```python
from build123d import *

# Parameters (mm, degrees)
SKIZZE1_W                       = 16
SKIZZE1_H                       = 63
SKIZZE6_W                       = 14.056140901
SKIZZE6_H                       = 6
SCHNITT_LINEAR_AUSTRAGEN2_DEPTH = 2.9
SKIZZE8_W                       = 9.697943534
SKIZZE8_H                       = 4.605462576
VERRUNDUNG1_R                   = 2.7
SKIZZE9_W                       = 13.512274764
SKIZZE9_H                       = 9
SKIZZE11_W                      = 2.793838278
SKIZZE11_H                      = 24.477994545
SKIZZE12_W                      = 8.586499361
SKIZZE12_H                      = 1
VERRUNDUNG2_R                   = 1.5
VERRUNDUNG3_R                   = 1
VERRUNDUNG4_R                   = 1


with BuildPart() as part:
    # Skizze1 → Rotation1 (revolve)
    with BuildSketch(Plane(origin=(0, 0, 0), x_dir=(0, 0, -1), z_dir=(1, 0, 0))):
        with Locations((-18, -0.15056419)):
            Rectangle(SKIZZE1_W, SKIZZE1_H)
    revolve(axis=Axis((0, 31.34943581, 10), (0, -1, 0)))

    # Skizze6 → Schnitt-Rotation1 (revolve, cut)
    with BuildSketch(Plane.XY.offset(10), mode=Mode.PRIVATE) as schnitt_rotation1_sk:
        with Locations((-10.028070451, 28.34943581)):
            Rectangle(SKIZZE6_W, SKIZZE6_H)
    revolve(schnitt_rotation1_sk.sketch.rotate(Axis((0, 55, 10), (0, -1, 0)), 270), axis=Axis((0, 55, 10), (0, -1, 0)), mode=Mode.SUBTRACT)

    # Skizze7 → Schnitt-Linear austragen2 (cut)
    with BuildSketch(Plane.XZ.offset(31.65056419)):
        with BuildLine():
            Line((-10.583005244, 22), (10.583005244, 22))
            ThreePointArc((10.583005244, 22), (0, 26), (-10.583005244, 22))
        make_face()
        with BuildLine():
            ThreePointArc((16, 10), (14.966629547, 15.656854249), (12, 20.583005244))
            Line((12, 20.583005244), (12, -0.583005244))
            ThreePointArc((12, -0.583005244), (14.966629547, 4.343145751), (16, 10))
        make_face()
        with BuildLine():
            ThreePointArc((-10.583005244, -2), (0, -6), (10.583005244, -2))
            Line((10.583005244, -2), (-10.583005244, -2))
        make_face()
        with BuildLine():
            Line((-12, -0.583005244), (-12, 20.583005244))
            ThreePointArc((-12, 20.583005244), (-16, 10), (-12, -0.583005244))
        make_face()
    extrude(amount=-SCHNITT_LINEAR_AUSTRAGEN2_DEPTH, mode=Mode.SUBTRACT)

    # Skizze8 → Schnitt-Rotation2 (revolve, cut)
    with BuildSketch(Plane.XY.offset(10), mode=Mode.PRIVATE) as schnitt_rotation2_sk:
        with Locations((-13.848971767, -26.447832902)):
            Rectangle(SKIZZE8_W, SKIZZE8_H)
    revolve(schnitt_rotation2_sk.sketch.rotate(Axis((0, 55, 10), (0, -1, 0)), 270), axis=Axis((0, 55, 10), (0, -1, 0)), mode=Mode.SUBTRACT)

    # Verrundung1
    # the kernel refuses this fillet: 2.7 mm, written as the material it takes off along each edge
    with BuildSketch(Plane(origin=(-12, -34.598571865, 20.583005244), x_dir=(0.6886261541674549, 0, 0.72511655600775), z_dir=(0, 1, 0)), Plane(origin=(-10.583005244, -34.598571865, -2), x_dir=(-0.7251165560077487, 0, 0.6886261541674565), z_dir=(0, 1, 0)), Plane(origin=(10.583005244, -34.598571865, 22), x_dir=(0.72511655600775, 0, -0.6886261541674551), z_dir=(0, 1, 0)), Plane(origin=(12, -34.598571865, -0.583005244), x_dir=(-0.6886261541674555, 0, -0.7251165560077496), z_dir=(0, 1, 0))) as verrundung1_piece_1:
        with BuildLine():
            CenterArc((1.079707811, 2.698166172), VERRUNDUNG1_R, 226.478544781, 45.633288329)
            Line((-0.779582805, 0.740351471), (0, 0))
            ThreePointArc((0, 0), (0.589601535, -0.010867127), (1.17920307, 0))
        make_face()
    extrude(amount=8.796015351, mode=Mode.SUBTRACT)
    with BuildSketch(Plane(origin=(-12, -34.598571865, -0.583005244), x_dir=(0, 0, 1), z_dir=(0, 1, 0)), Plane(origin=(10.583005244, -34.598571865, -2), x_dir=(-1, 0, 0), z_dir=(0, 1, 0)), Plane(origin=(12, -34.598571865, 20.583005244), x_dir=(0, 0, -1), z_dir=(0, 1, 0))) as verrundung1_piece_2:
        with BuildLine():
            CenterArc((1.075113785, 2.7), VERRUNDUNG1_R, 224.366711671, 45.633288329)
            ThreePointArc((-0.855059669, 0.812030075), (-0.435013222, 0.398135104), (0, 0))
            Line((0, 0), (1.075113785, 0))
        make_face()
    extrude(amount=8.796015351, mode=Mode.SUBTRACT)
    with BuildSketch(Plane(origin=(-10.583005244, -34.598571865, 22), x_dir=(-0.7251165560077509, 0, -0.6886261541674541), z_dir=(0, 1, 0))) as verrundung1_piece_3:
        with BuildLine():
            CenterArc((1.079707811, -2.698166172), VERRUNDUNG1_R, 87.88816689, 45.633288329)
            Line((-0.779582805, -0.740351471), (0, 0))
            ThreePointArc((0, 0), (0.589601535, 0.010867127), (1.17920307, 0))
        make_face()
    extrude(amount=8.796015351, mode=Mode.SUBTRACT)

    # Skizze9 → Schnitt-Rotation3 (revolve, cut)
    with BuildSketch(Plane.XY.offset(10), mode=Mode.PRIVATE) as schnitt_rotation3_sk:
        with Locations((10.756137382, 11.84943581)):
            Rectangle(SKIZZE9_W, SKIZZE9_H)
    revolve(schnitt_rotation3_sk.sketch.rotate(Axis((0, 55, 10), (0, -1, 0)), 90), axis=Axis((0, 55, 10), (0, -1, 0)), mode=Mode.SUBTRACT)

    # Skizze11 → Schnitt-Rotation4 (revolve, cut)
    with BuildSketch(Plane.XY.offset(10), mode=Mode.PRIVATE) as schnitt_rotation4_sk:
        with Locations((-16.396919139, -4.411566918)):
            Rectangle(SKIZZE11_W, SKIZZE11_H)
    revolve(schnitt_rotation4_sk.sketch.rotate(Axis((0, 55, 10), (0, -1, 0)), 270), axis=Axis((0, 55, 10), (0, -1, 0)), mode=Mode.SUBTRACT)

    # Skizze12 → Schnitt-Rotation5 (revolve, cut)
    with BuildSketch(Plane.XY.offset(10), mode=Mode.PRIVATE) as schnitt_rotation5_sk:
        with Locations((-13.293249681, -16.15056419)):
            Rectangle(SKIZZE12_W, SKIZZE12_H)
    revolve(schnitt_rotation5_sk.sketch.rotate(Axis((0, 55, 10), (0, -1, 0)), 270), axis=Axis((0, 55, 10), (0, -1, 0)), mode=Mode.SUBTRACT)

    # Verrundung2
    verrundung2_edges = [part.edges().sort_by_distance(p)[0] for p in [
        (0, 25.34943581, -6),
    ]]
    fillet(verrundung2_edges, radius=VERRUNDUNG2_R)

    # Verrundung3
    verrundung3_edges = [part.edges().sort_by_distance(p)[0] for p in [
        (0, -16.65056419, -6),
        (0, -24.145101614, -6),
    ]]
    fillet(verrundung3_edges, radius=VERRUNDUNG3_R)

    # Verrundung4
    verrundung4_edges = [part.edges().sort_by_distance(p)[0] for p in [
        (0, 7.34943581, -5),
        (0, -15.65056419, -5),
    ]]
    fillet(verrundung4_edges, radius=VERRUNDUNG4_R)


solid = part.part
```
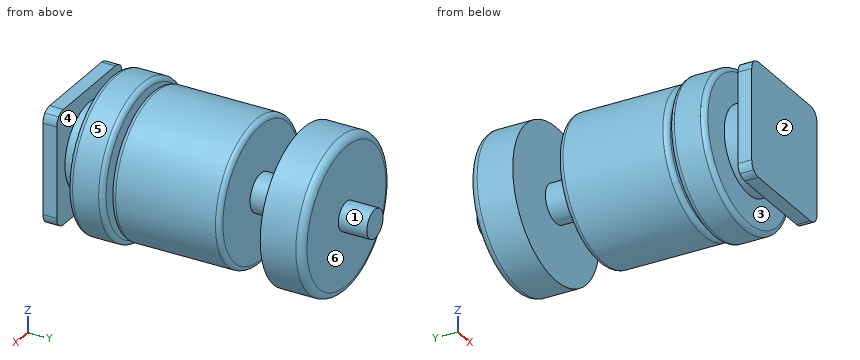
For this review, take the finished solid that the model builds, in its own axes (mm). Face numbers are marked on the shaded views. A direction names the side the tool comes from. Give positions to 0.01 mm unless a question says otherwise; leave off trailing zeros. Write each loop counter-clockwise with the first axis right and the second up, starting at its lowest first coordinate (ties: lowest second). Pieces come first, ordered by that corner, then holes. Notation, with made-up numbers: M 38,55 L 83,55 A36 cw 83,94 Z; hole C 60,29.5 d8. An arc over 180 degrees is marked long. Answer as a JSON object with one key per item and string values. Group by question number.
Item 1: Consider section A-A on y = -13. Write out the cut boundary in (x, z).
Item 2: Tool access review of the marked faces 1, 2 and 3: name each direction out of +Z, -Z, +X, -X, +Y, -Y from which nothing blocks a thin tool from reaching the whole face with its end or side.
Item 3: Consider section B-B on y = 19. Write out the cut boundary in (x, z).
Item 4: Draft analysis for pull direction Y (two halves, no side actions). For the marked faces 4, 5 and 6, state which applies: +Y half, -Y half, draft (parallel to the pull), parting line (faces both ways), or undercut.
Item 5: For pin 1 Ø2.5 at (x, y) = (0.5, -31) entering from -Z; pin 2 Ø1.4 at (y, z) = (-30.5, 11.5) entering from -X; pin 3 Ø3 at (x, y) = (1, -30.5) entering from +Z, all flat-tipped, find the tip position at first contact; note any pin that passes through.
Item 6: For probe 1 along Y at (x, z) = (-11, 7.5); probe 2 along Y at (x, z) = (3.5, -3); probe 3 along Y at (x, z) = (-5, 10), list the stretches that pass through material, from the lowest coordinate up. Write a range as [from, to].
Check result:
{
 "1": {"outline": "C 0,10 d30"},
 "2": {"face 1": "+Y", "face 2": "+Z, -Z, +X, -X, -Y", "face 3": "none"},
 "3": {"outline": "C 0,10 d32"},
 "4": {"face 4": "undercut", "face 5": "draft", "face 6": "+Y half"},
 "5": {"pin 1": "stops at z = -2", "pin 2": "stops at x = -12", "pin 3": "stops at z = 22"},
 "6": {"probe 1": "y = [-31.65, -28.75], [-24.15, -16.65], [-15.65, 7.35], [16.35, 25.35]", "probe 2": "y = [-24.15, -16.65], [-15.65, 7.35], [16.35, 25.35]", "probe 3": "y = [-31.65, 7.35], [16.35, 25.35]"}
}
